The figure shows three views and two pictorial views of one solid part (mm, origin at its lowest corner). Answer the questions. A direction names the side the tool comes from. Give positions to 0.01 mm unless a question says otherwise; leave off trailing zeros. Loops run counter-clockwise (first coordinate to the right, second up) from the corner with the lowest first, then second, coordinate; pieces in that order, holes last.
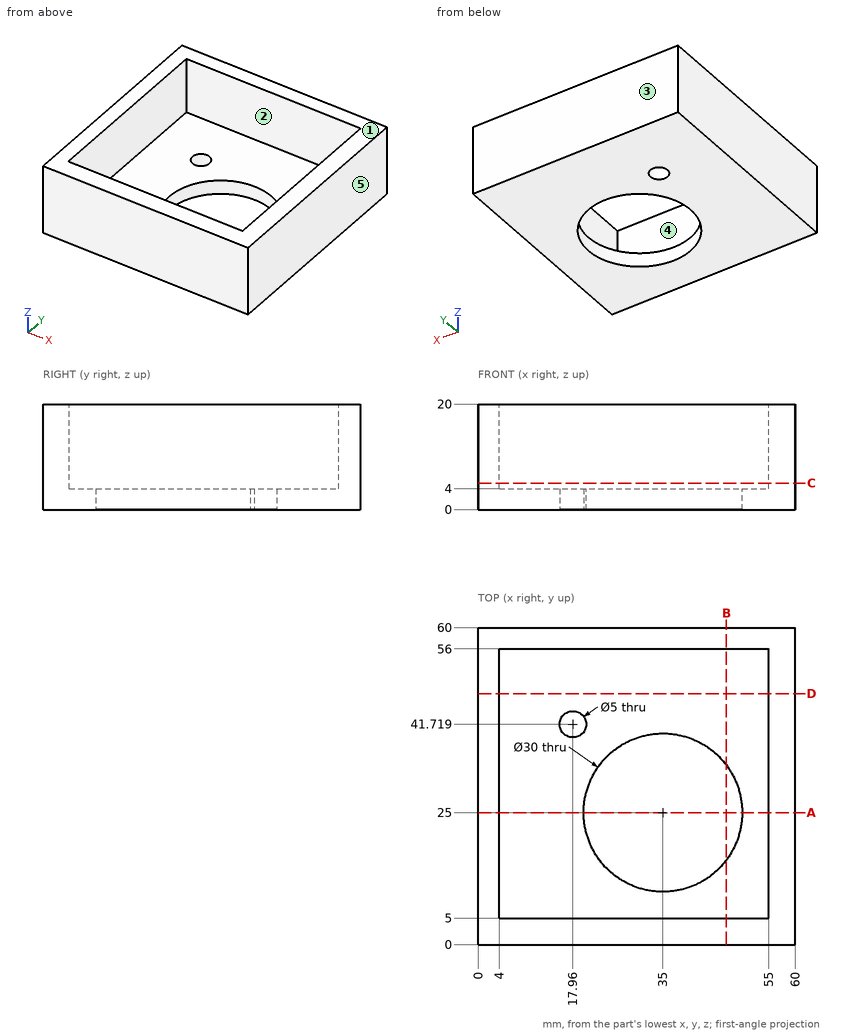
Q1. Determine the mould class of the marked faces 3, 4 and 5 for opening direction X: +X half, -X half, draft (parallel to the pull), parting line (faces both ways), or undercut.
Q2. Section D-D on y = 47.5 is taken. Give the vertices of the cut face in (x, z), plus the area to 3 significant figures.
Q3. Section A-A on y = 25 is taken. Give the vertices of the cut face in (x, z), plus the area to 3 significant figures.
Q4. Section C-C on z = 5 is taken. Give the vertices of the cut face in (x, y), plus the area to 3 significant figures.
Q5. Consider line 1 along Y through (x, z) = (54, 9); line 2 along Y through (x, z) = (35, 1.2); line 3 along X through (y, z) = (26, 9.25). Determine where each line is inside the solid, lowest interval first.
Q6. Which of the six approach directions +Z, -Z, +X, -X, +Y, -Y give full straight-line access (tool end or side, diameter ignored) to the marked faces 1 and 2?
Q7. Given pin 1 (4 mm diameter, centred on x = 17.96, y = 41.72, fed in from +Z), flat-ended and moving along its own axis, determine where the tip first touches the part or whether it passes through.
Q8. Section B-B on x = 47 is taken. Give the vertices of the cut face in (y, z), plus the area to 3 significant figures.
Check result:
1. face 3: draft
1. face 4: undercut
1. face 5: +X half
2. outline: (0, 0) - (60, 0) - (60, 20) - (55, 20) - (55, 4) - (4, 4) - (4, 20) - (0, 20) - close
2. area: 384 mm2
3. outline: (0, 0) - (20, 0) - (20, 4) - (4, 4) - (4, 20) - (0, 20) - close; (50, 0) - (60, 0) - (60, 20) - (55, 20) - (55, 4) - (50, 4) - close
3. area: 264 mm2
4. outline: (0, 0) - (60, 0) - (60, 60) - (0, 60) - close; hole (4, 5) - (55, 5) - (55, 56) - (4, 56) - close
4. area: 999 mm2
5. line 1: y = 0 to 5, 56 to 60
5. line 2: y = 0 to 10, 40 to 60
5. line 3: x = 0 to 4, 55 to 60
6. face 1: +Z, +X, -X, +Y, -Y
6. face 2: +Z
7. pin 1: passes through
8. outline: (0, 0) - (16, 0) - (16, 4) - (5, 4) - (5, 20) - (0, 20) - close; (34, 0) - (60, 0) - (60, 20) - (56, 20) - (56, 4) - (34, 4) - close
8. area: 312 mm2
